Geometry check sheet. Reference: the model listing, model coordinates, mm. Face numbers are marked on the shaded views. A direction names the side the tool comes from. Give positions to 0.01 mm unless a question says otherwise; leave off trailing zeros. Order: outer loops, then holes, each group sorted by start corner. A loop starts at its lowest first (then second) coordinate and runs counter-clockwise, first axis right, second up. Notation, with made-up numbers: (4, 31.5) - (47, 31.5) arc R17 cw to (47, 57.5) - close; hole circle Ø4 at (72, 73.5). An arc over 180 degrees is marked (long way). Put each result on its own line as item: value. Start each with the question number.
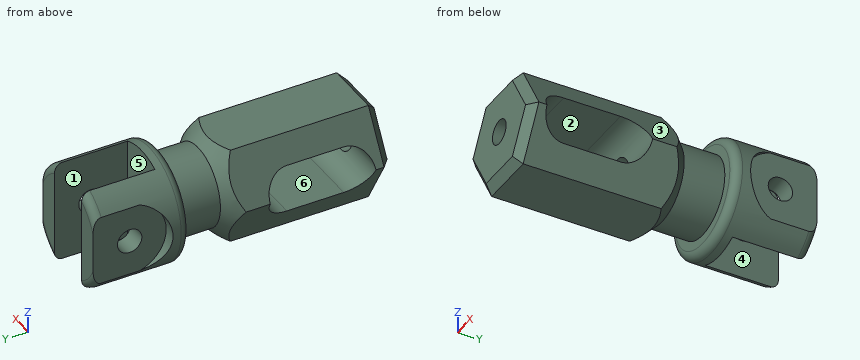
```python
from build123d import *

# Parameters (mm, degrees)
BOSS_EXTRUDE1_DEPTH     = 100
CHAMFER1_SIZE           = 5
CUT_EXTRUDE1_DEPTH      = 35.641016151
CUT_EXTRUDE1_DEPTH_BACK = 35.641016151
SKETCH3_R               = 24.5
BOSS_EXTRUDE2_DEPTH     = 25
SKETCH5_R               = 35
BOSS_EXTRUDE3_DEPTH     = 55
FILLET1_R               = 5
SKETCH6_W               = 30
SKETCH6_H               = 45
CUT_EXTRUDE2_DEPTH      = 36.0000001
CUT_EXTRUDE2_DEPTH_BACK = 36.0000001
CUT_EXTRUDE3_DEPTH      = 8.5
SKETCH8_R               = 7.5
CUT_EXTRUDE4_DEPTH      = 55
FILLET2_R               = 5
SKETCH9_R               = 7.5
CUT_EXTRUDE5_DEPTH      = 181.0000001


with BuildPart() as part:
    # Sketch1 → Boss-Extrude1 (new body)
    with BuildSketch(Plane(origin=(0, 0, 0), x_dir=(1, 0, 0), z_dir=(0, 1, 0))):
        Polygon((34.641016151, 0), (17.320508076, 30), (-17.320508076, 30), (-34.641016151, 0), (-17.320508076, -30), (17.320508076, -30), align=None)
    extrude(amount=BOSS_EXTRUDE1_DEPTH)

    # Chamfer1
    chamfer1_edges = [part.edges().sort_by_distance(p)[0] for p in [
        (0, 0, 30),
        (-25.980762114, 0, 15),
        (-25.980762114, 0, -15),
        (0, 0, -30),
        (25.980762114, 0, -15),
        (25.980762114, 0, 15),
    ]]
    chamfer(chamfer1_edges, length=CHAMFER1_SIZE)

    # Sketch2 → Cut-Extrude1 (cut, two sides)
    with BuildSketch(Plane(origin=(0, 0, 0), x_dir=(0, 0, -1), z_dir=(1, 0, 0))) as cut_extrude1_sk:
        with BuildLine():
            Line((15, 60), (15, 25))
            ThreePointArc((15, 25), (0, 10), (-15, 25))
            Line((-15, 25), (-15, 60))
            ThreePointArc((-15, 60), (0, 75), (15, 60))
        make_face()
    extrude(amount=CUT_EXTRUDE1_DEPTH, mode=Mode.SUBTRACT)
    extrude(cut_extrude1_sk.sketch, amount=-CUT_EXTRUDE1_DEPTH_BACK, mode=Mode.SUBTRACT)

    # Sketch3 → Boss-Extrude2 (add)
    with BuildSketch(Plane(origin=(0, 100, 0), x_dir=(1, 0, 0), z_dir=(0, 1, 0))):
        Circle(SKETCH3_R)
    extrude(amount=BOSS_EXTRUDE2_DEPTH)

    # Sketch4 → Cut-Revolve1 (revolve, cut)
    with BuildSketch(Plane.XY):
        Polygon((-24.5, 100), (-37.5, 87), (-37.5, 100), align=None)
    revolve(axis=Axis((0, -6.25, 0), (0, 1, 0)), mode=Mode.SUBTRACT)

    # Sketch5 → Boss-Extrude3 (add)
    with BuildSketch(Plane(origin=(0, 125, 0), x_dir=(1, 0, 0), z_dir=(0, 1, 0))):
        Circle(SKETCH5_R)
    extrude(amount=BOSS_EXTRUDE3_DEPTH)

    # Fillet1
    fillet1_edges = [part.edges().sort_by_distance(p)[0] for p in [
        (-35, 125, 0),
    ]]
    fillet(fillet1_edges, radius=FILLET1_R)

    # Sketch6 → Cut-Extrude2 (cut, two sides)
    with BuildSketch(Plane.XY) as cut_extrude2_sk:
        with Locations((0, 157.5)):
            Rectangle(SKETCH6_W, SKETCH6_H)
    extrude(amount=CUT_EXTRUDE2_DEPTH, mode=Mode.SUBTRACT)
    extrude(cut_extrude2_sk.sketch, amount=-CUT_EXTRUDE2_DEPTH_BACK, mode=Mode.SUBTRACT)

    # Sketch7 → Cut-Extrude3 (cut, through all)
    with BuildSketch(Plane(origin=(27.5, 0, 0), x_dir=(0, 0, -1), z_dir=(1, 0, 0))):
        with BuildLine():
            Line((-22.5, 180), (22.5, 180))
            Line((22.5, 180), (22.5, 157.5))
            ThreePointArc((22.5, 157.5), (0, 135), (-22.5, 157.5))
            Line((-22.5, 157.5), (-22.5, 180))
        make_face()
    cut_extrude3 = extrude(amount=CUT_EXTRUDE3_DEPTH, mode=Mode.SUBTRACT)

    # Mirror1: Cut-Extrude3 across plane
    add(cut_extrude3.mirror(Plane(origin=(0, 0, 0), x_dir=(0, 0, 1), z_dir=(1, 0, 0))), mode=Mode.SUBTRACT)

    # Sketch8 → Cut-Extrude4 (cut)
    with BuildSketch(Plane(origin=(27.5, 0, 0), x_dir=(0, 0, -1), z_dir=(1, 0, 0))):
        with Locations((0, 157.5)):
            Circle(SKETCH8_R)
    extrude(amount=-CUT_EXTRUDE4_DEPTH, mode=Mode.SUBTRACT)

    # Fillet2
    fillet2_edges = [part.edges().sort_by_distance(p)[0] for p in [
        (21.827125362, 180, -27.360127895),
        (-21.827125362, 180, 27.360127895),
        (21.827125362, 180, 27.360127895),
        (-21.827125362, 180, -27.360127895),
    ]]
    fillet(fillet2_edges, radius=FILLET2_R)

    # Sketch9 → Cut-Extrude5 (cut, through all)
    with BuildSketch(Plane.XZ):
        Circle(SKETCH9_R)
    extrude(amount=-CUT_EXTRUDE5_DEPTH, mode=Mode.SUBTRACT)


solid = part.part
```
Item 1: Cross-section at B-B (x = 0). Enter the section's corners in (y, z).
Item 2: Cross-section at C-C (y = 39). Enter the section's corners in (x, z), and give its area (3 significant figures).
Item 3: Cross-section at A-A (y = 157.5). Enter the section's corners in (x, z).
Item 4: Cross-section at D-D (y = 83). Enter the section's corners in (x, z).
Item 5: Set-up check for the marked faces 1, 2 and 3: record each of +Z, -Z, +X, -X, +Y, -Y from which the full face is reachable in a straight line by a thin tool's end or side.
Item 6: Release check for a two-part mould opening along Y. For the marked faces 4, 5 and 6 record: +Y half, -Y half, draft (parallel to the pull), parting line (faces both ways), or undercut.
Item 7: Thickness scan on line 1 along Z through (x, y) = (-5.5, 56); line 2 along Z through (x, y) = (0, 6.5); line 3 along X through (y, z) = (109, 0). Record the ranges inside material, lowest first.
Item 8: Gauge pin test, flat ends, axial feed: pin 1 Ø10.5 at (x, y) = (-10, 48) entering from +Z; pin 2 Ø21.5 at (y, z) = (160.5, -2.5) entering from -X; pin 3 Ø13.5 at (y, z) = (168, -15) entering from +X. Record the tip position at first contact, or that the pin passes through.
Recorded:
1. outline: (0, -25) - (5, -30) - (94.5, -30) - (100, -24.5) - (125, -24.5) - (125, -30) arc R5 ccw to (130, -35) - (135, -35) - (135, -7.5) - (72.99, -7.5) arc R15 cw to (60, -15) - (25, -15) arc R15 cw to (12.01, -7.5) - (0, -7.5) - close; (0, 7.5) - (12.01, 7.5) arc R15 cw to (25, 15) - (60, 15) arc R15 cw to (72.99, 7.5) - (135, 7.5) - (135, 35) - (130, 35) arc R5 ccw to (125, 30) - (125, 24.5) - (100, 24.5) - (94.5, 30) - (5, 30) - (0, 25) - close
2. outline: (-25.98, -15) - (-17.32, -30) - (17.32, -30) - (25.98, -15) - close; (-25.98, 15) - (25.98, 15) - (17.32, 30) - (-17.32, 30) - close
2. area: 1,300 mm^2
3. outline: (-27.5, -21.65) arc R35 ccw to (-15, -31.62) - (-15, -7.5) - (-27.5, -7.5) - close; (-27.5, 7.5) - (-15, 7.5) - (-15, 31.62) arc R35 ccw to (-27.5, 21.65) - close; (15, -31.62) arc R35 ccw to (27.5, -21.65) - (27.5, -7.5) - (15, -7.5) - close; (15, 7.5) - (27.5, 7.5) - (27.5, 21.65) arc R35 ccw to (15, 31.62) - close
4. outline: (-34.64, 0) - (-17.32, -30) - (17.32, -30) - (34.64, 0) - (17.32, 30) - (-17.32, 30) - close; hole circle Ø15 at (0, 0)
5. face 1: +Z, -Z, +Y
5. face 2: +X, -X
5. face 3: +Z, +X, -Y
6. face 4: draft
6. face 5: +Y half
6. face 6: undercut
7. line 1: z = -30 to -15, 15 to 30
7. line 2: z = -30 to -7.5, 7.5 to 30
7. line 3: x = -24.5 to -7.5, 7.5 to 24.5
8. pin 1: stops at z = 30
8. pin 2: stops at x = -27.5
8. pin 3: stops at x = 27.5
